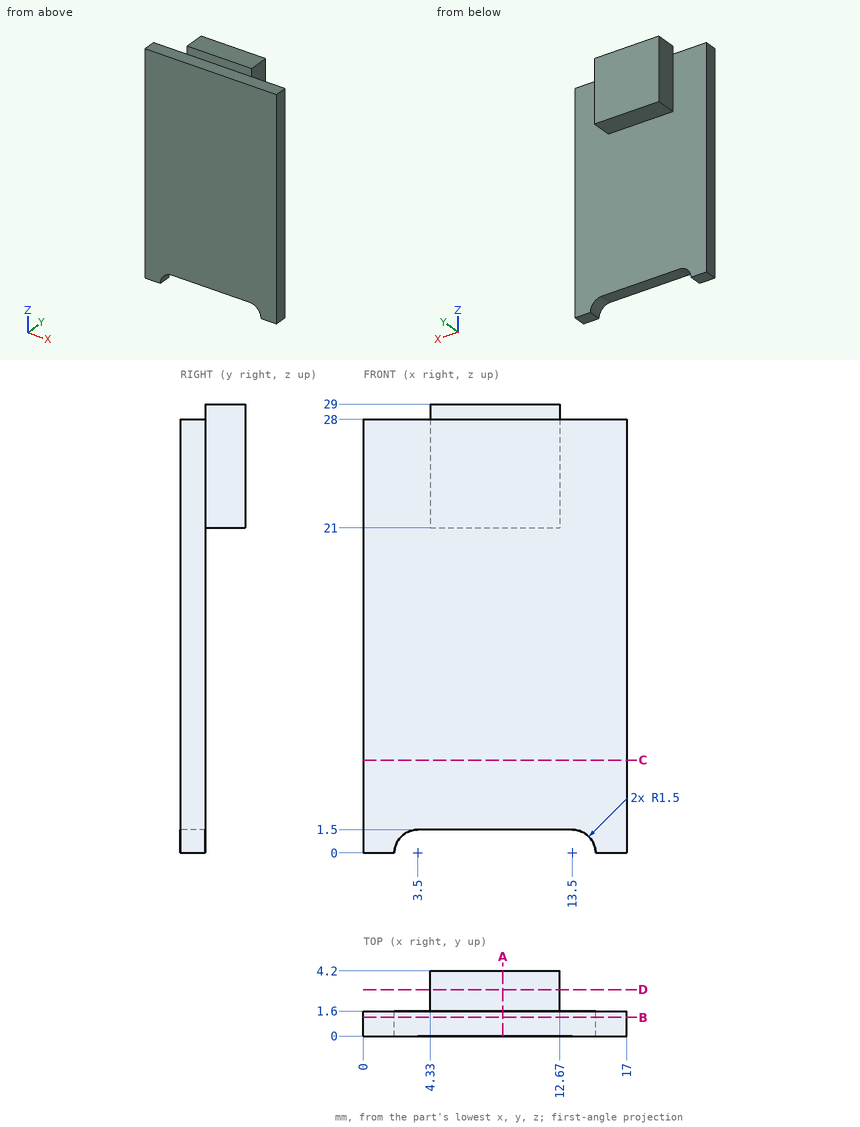
For this review, use the dimensioned drawing (mm, ordinates from the lowest corner) and the shaded views. Give positions to 0.01 mm unless a question says otherwise; leave off trailing zeros. Loops run counter-clockwise (first coordinate to the right, second up) from the corner with the lowest first, then second, coordinate; pieces in that order, holes last. Notation, with made-up numbers: (14.5, -34) -> (62.5, -34) arc R13 cw to (62.5, -26) -> close; hole circle Ø9 at (59, 65). An arc over 180 degrees is marked (long way). Use CSV: the item, a comma, the result in double quotes.
1. Consider section B-B, the plane y = 1.2. Write out the cut boundary in (x, z).
Result:
outline,"(0, 0) -> (2, 0) arc R1.5 cw to (3.5, 1.5) -> (13.5, 1.5) arc R1.5 cw to (15, 0) -> (17, 0) -> (17, 28) -> (0, 28) -> close"
2. Consider section A-A, the plane x = 9. Write out the cut boundary in (y, z).
Result:
outline,"(0, 1.5) -> (1.6, 1.5) -> (1.6, 21) -> (4.2, 21) -> (4.2, 29) -> (1.6, 29) -> (1.6, 28) -> (0, 28) -> close"
3. Consider section D-D, the plane y = 3. Write out the cut boundary in (x, z).
Result:
outline,"(4.33, 21) -> (12.67, 21) -> (12.67, 29) -> (4.33, 29) -> close"
4. Consider section C-C, the plane z = 6. Write out the cut boundary in (x, y).
Result:
outline,"(0, 0) -> (17, 0) -> (17, 1.6) -> (0, 1.6) -> close"
5. To check wall thickness, follow probe 1 along Y at (x, z) = (13.5, 20.25); probe 2 along Z at (x, y) = (16.5, 1.25); probe 3 along X at (y, z) = (2.5, 26.5). State the ranges of each line that lie inside material, in increasing order. Write a range as from..to.
Result:
probe 1,"y = 0..1.6"
probe 2,"z = 0..28"
probe 3,"x = 4.33..12.67"
6. For P1, Ø1.5, axis at y = 1, z = 11, coming from the -X side; P2, Ø8, axis at x = 8, z = 16, coming from the +Y side; P3, Ø1.3, axis at y = 2.5, z = 24, coming from the -X side; P4, Ø1.3, axis at x = 8.5, y = 3, coming from the -Z side, all flat-tipped, find the tip position at first contact; note any pin that passes through.
Result:
P1,"stops at x = 0"
P2,"stops at y = 1.6"
P3,"stops at x = 4.33"
P4,"stops at z = 21"
